Design review of the part shown in the three views and the two pictorial views. Dimensions are in mm from the part's minimum x, y and z. Coordinates: 2 decimals unless noted, no trailing zeros. Loops run counter-clockwise (first coordinate to the right, second up) from the corner with the lowest first, then second, coordinate; pieces in that order, holes last.
Q1. Add section A-A on y = 1.1. Give the boundary of the cut face in (x, z) (1 decimal), and give its area (3 significant figures).
Q2. Add section D-D on z = 8. Give the boundary of the cut face in (x, y) (1 decimal).
Q3. Add section C-C on z = 1.75. Give the boundary of the cut face in (x, y) (1 decimal).
Q4. Wall thickness on probe 1 along X at (y, z) = (0.35, 4.5) (1 decimal); probe 2 along X at (y, z) = (0.3, 4.25) (1 decimal); probe 3 along X at (y, z) = (1.5, 6.5) (1 decimal): over which ranges is each line inside the solid? List them lowest first.
Q5. Add section B-B on x = 50. Give the boundary of the cut face in (y, z) (1 decimal).
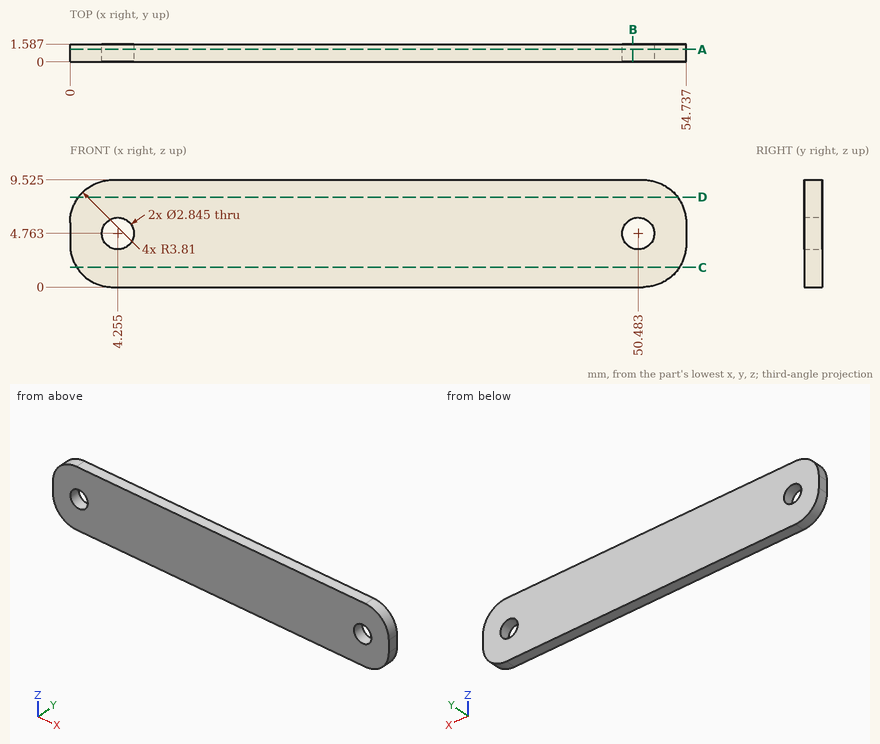
Entries:
1. outline: (0, 3.8) arc R3.8 ccw to (3.8, 0) - (50.9, 0) arc R3.8 ccw to (54.7, 3.8) - (54.7, 5.7) arc R3.8 ccw to (50.9, 9.5) - (3.8, 9.5) arc R3.8 ccw to (0, 5.7) - close; hole circle Ø2.8 at (4.3, 4.8); hole circle Ø2.8 at (50.5, 4.8)
1. area: 496 mm2
2. outline: (0.8, 0) - (54, 0) - (54, 1.6) - (0.8, 1.6) - close
3. outline: (0.6, 0) - (54.1, 0) - (54.1, 1.6) - (0.6, 1.6) - close
4. probe 1: x = 0 to 2.9, 5.7 to 49.1, 51.9 to 54.7
4. probe 2: x = 0 to 2.9, 5.6 to 49.2, 51.8 to 54.7
4. probe 3: x = 0.1 to 54.7
5. outline: (0, 0) - (1.6, 0) - (1.6, 3.4) - (0, 3.4) - close; (0, 6.1) - (1.6, 6.1) - (1.6, 9.5) - (0, 9.5) - close
